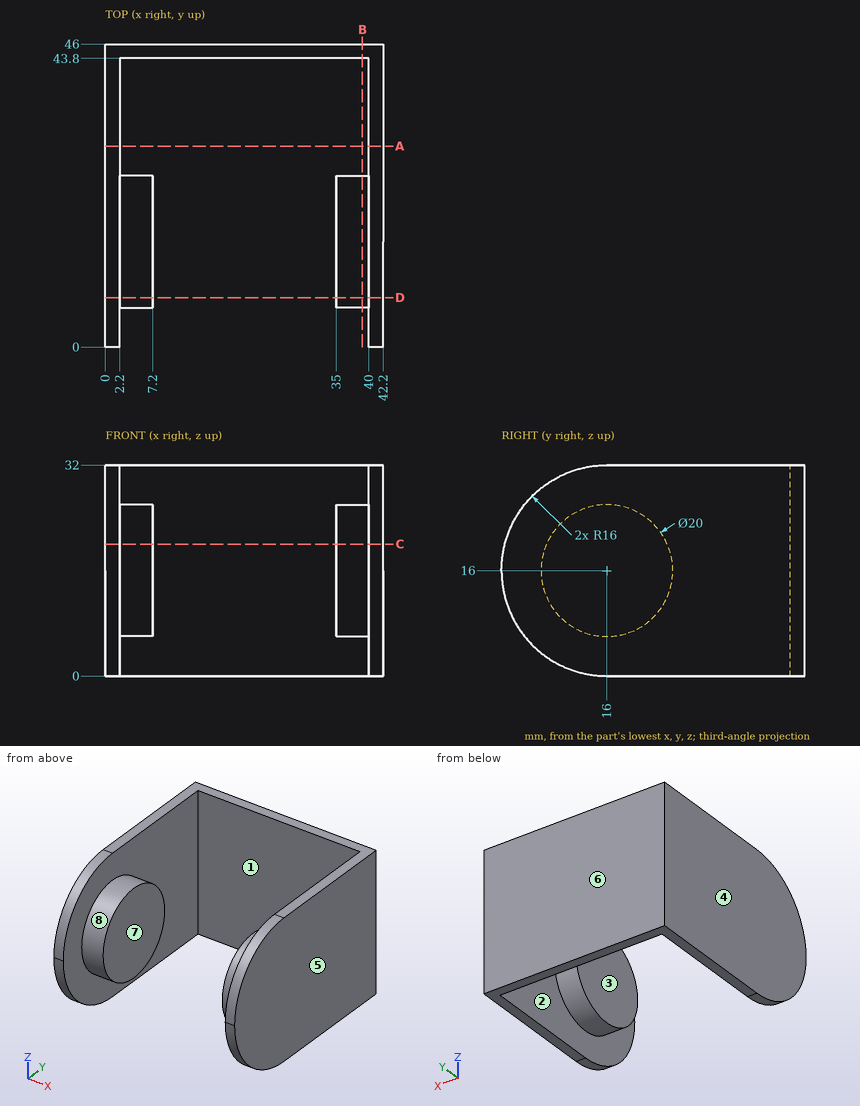
Check sheet for the drawn part. Datum: minimum x, y, z corner. Units: mm. A direction names the side the tool comes from. Give positions to 0.01 mm unless a question says otherwise; leave off trailing zeros. Loops run counter-clockwise (first coordinate to the right, second up) from the corner with the lowest first, then second, coordinate; pieces in that order, holes last. Notation, with made-up numbers: M 89,-23 L 97,-23 A17 ccw 97,-8 Z; hole C -15.5,13.5 d11. An arc over 180 degrees is marked long. Return JSON: item names as keys, results as strings.
1) Tool access check on the marked faces 1, 2, 3 and 4. Record the directions out of +Z, -Z, +X, -X, +Y, -Y that give a thin tool (end or side, any length) a straight path to the whole face; none if there is none.
Findings:
{"face 1": "+Z, -Z", "face 2": "none", "face 3": "+Z, -Z, -Y", "face 4": "+Z, -Z, -X, +Y, -Y"}
2) Mould release check, pull along X, two halves, no side actions. Record for the marked faces 5, 6, 7 and 8: released by +X, released by -X, zero draft, split by the parting line, or undercut.
Findings:
{"face 5": "released by +X", "face 6": "zero draft", "face 7": "undercut", "face 8": "undercut"}
3) Section check C-C, the plane z = 20. Enter the section's corners in (x, y) (3 decimals), and give its area (3 significant figures).
Findings:
{"outline": "M 0,0.508 L 2.2,0.508 L 2.2,6.835 L 7.2,6.835 L 7.2,25.165 L 2.2,25.165 L 2.2,43.8 L 40,43.8 L 40,25.165 L 35,25.165 L 35,6.835 L 40,6.835 L 40,0.508 L 42.2,0.508 L 42.2,46 L 0,46 Z", "area": "467 mm2"}
4) Section check B-B, the plane x = 39. Enter the section's corners in (y, z), and give its area (3 significant figures).
Findings:
{"outline": "C 16,16 d20; M 43.8,0 L 46,0 L 46,32 L 43.8,32 Z", "area": "385 mm2"}
5) Section check D-D, the plane y = 7.5. Enter the section's corners in (x, z).
Findings:
{"outline": "M 0,2.44 L 2.2,2.44 L 2.2,10.73 L 7.2,10.73 L 7.2,21.27 L 2.2,21.27 L 2.2,29.56 L 0,29.56 Z; M 35,10.73 L 40,10.73 L 40,2.44 L 42.2,2.44 L 42.2,29.56 L 40,29.56 L 40,21.27 L 35,21.27 Z"}
6) Gauge pin test, flat end, axial feed: P1, Ø1, axis at x = 28.5, z = 8, coming from the -Y side. Record the tip position at first contact, or that the pin passes through.
Findings:
{"P1": "stops at y = 43.8"}
7) Section check A-A, the plane y = 30.5. Enter the section's corners in (x, z).
Findings:
{"outline": "M 0,0 L 2.2,0 L 2.2,32 L 0,32 Z; M 40,0 L 42.2,0 L 42.2,32 L 40,32 Z"}
8) Material ranges on L1, parallel to X at y = 17, z = 13.5; L2, parallel to X at y = 32, z = 9.5; L3, parallel to Y at x = 10.5, z = 30, recorded low to high. Write a range as [from, to].
Findings:
{"L1": "x = [0, 7.2], [35, 42.2]", "L2": "x = [0, 2.2], [40, 42.2]", "L3": "y = [43.8, 46]"}
